For this review, take the finished solid that the model builds, in its own axes (mm). A direction names the side the tool comes from. Give positions to 0.01 mm unless a question says otherwise; leave off trailing zeros. Loops run counter-clockwise (first coordinate to the right, second up) from the corner with the lowest first, then second, coordinate; pieces in that order, holes last. Notation, with made-up numbers: (-9.5, 65) -> (19.5, 65) arc R18 cw to (19.5, 91) -> close; hole circle Ø5 at (58, -4.5). An arc over 180 degrees is marked (long way). Write each question's results on one line, items separated by ' | '. Start each with the question number.
```python
from build123d import *

# Parameters (mm, degrees)
SKETCH_R          = 2
PAD_DEPTH         = 26
POCKET_DEPTH      = 12
POCKET_DEPTH_BACK = -12
POCKET001_DEPTH   = 4
CHAMFER_SIZE      = 3
SKETCH003_R       = 3
POCKET002_DEPTH   = 26
SKETCH004_R       = 6.75
POCKET003_DEPTH   = 5
FILLET_R          = 4.5
FILLET001_R       = 5
CHAMFER001_SIZE   = 0.5


with BuildPart() as part:
    # Sketch → Pad (new body)
    with BuildSketch(Plane.XY):
        with BuildLine():
            ThreePointArc((1e-06, -3.5), (3.416335, -0.760696), (1.485025, 3.169337))
            Line((-45.1066, 25), (1.485025, 3.169337))
            Line((-45.1066, 7.106602), (-45.1066, 25))
            Line((-34.499999, -3.5), (-45.1066, 7.106602))
            Line((1e-06, -3.5), (-34.499999, -3.5))
        make_face()
        Circle(SKETCH_R, mode=Mode.SUBTRACT)
    extrude(amount=PAD_DEPTH)

    # Sketch001 (on DatumPlane) → Pocket (cut, two sides)
    with BuildSketch(Plane.XY.offset(13)) as pocket_sk:
        Polygon((-60, 17), (-10, 17), (-60, 55), align=None)
    extrude(amount=-POCKET_DEPTH, mode=Mode.SUBTRACT)
    extrude(pocket_sk.sketch, amount=-POCKET_DEPTH_BACK, mode=Mode.SUBTRACT)

    # Sketch002 → Pocket001 (cut)
    with BuildSketch(Plane.XY):
        Polygon((-19.5, -3.5), (-30.106602, 7.106602), (-45.106602, 7.106602), (-34.5, -3.5), align=None)
    extrude(amount=POCKET001_DEPTH, mode=Mode.SUBTRACT)

    # Chamfer
    chamfer_edges = [part.edges().sort_by_distance(p)[0] for p in [
        (-36.569686, 17, 1),
        (-36.569686, 17, 25),
    ]]
    chamfer(chamfer_edges, length=CHAMFER_SIZE)

    # Sketch003 → Pocket002 (cut)
    with BuildSketch(Plane.XY):
        with Locations((-32.5, 1.5)):
            Circle(SKETCH003_R)
    extrude(amount=POCKET002_DEPTH, mode=Mode.SUBTRACT)

    # Sketch004 → Pocket003 (cut)
    with BuildSketch(Plane.XZ):
        with Locations((-20, 13)):
            Circle(SKETCH004_R)
    extrude(amount=POCKET003_DEPTH, mode=Mode.SUBTRACT)

    # Fillet
    fillet_edges = [part.edges().sort_by_distance(p)[0] for p in [
        (-45.1066, 17, 13),
        (-45.1066, 18.5, 2.5),
        (-45.1066, 18.5, 23.5),
        (-31.234114, 18.5, 23.5),
        (-31.234114, 18.5, 2.5),
    ]]
    fillet(fillet_edges, radius=FILLET_R)

    # Fillet001
    fillet001_edges = [part.edges().sort_by_distance(p)[0] for p in [
        (-45.1066, 25, 0.5),
        (-45.1066, 25, 25.5),
    ]]
    fillet(fillet001_edges, radius=FILLET001_R)

    # Chamfer001
    chamfer001_edges = [part.edges().sort_by_distance(p)[0] for p in [
        (-39.803299, 1.803301, 26),
        (-18.250068, 12.416282, 26),
    ]]
    chamfer(chamfer001_edges, length=CHAMFER001_SIZE)


solid = part.part
```
1. We need section A-A (x = -1). Write out the cut boundary in (y, z).
2. For pin 1 Ø10 at (x, z) = (-34, 10.5) entering from +Y; pin 2 Ø5 at (y, z) = (17, 19.5) entering from +X; pin 3 Ø10 at (y, z) = (9, 4) entering from +X, all flat-tipped, find the tip position at first contact; note any pin that passes through.
3. We need section C-C (x = -20). Write out the cut boundary in (y, z).
4. We need section D-D (y = 10.5). Write out the cut boundary in (x, z), plus the area to 3 significant figures.
5. We need section B-B (z = 21.5). Write out the cut boundary in (x, y).
6. Wall thickness on L1, parallel to Z at x = -20, y = -2.75; L2, parallel to Y at x = -32.5, z = 10; L3, parallel to X at y = -1.75, z = 8.25: over which ranges is each line inside the solid? List them lowest first.
7. Machinability: for faces 4 (the flat face through (-39.55, 1.9, 25.75)), 5 (the cylindrical face through (-43.82, 15.65, 12.85)), 6 (the flat face through (-37, 18, 23)), 7 (the flat face through (-29.6, 3.1, 4)), 8 (the cylindrical face through (-42.73, 21.39, 0.51)), which of the approach directions +Z, -Z, +X, -X, +Y, -Y give a long, thin tool a straight path to every point of the face, cutting with its end or side? Answer none if there is none.
8. Draft analysis for pull direction X (two halves, no side actions). For faces 1 (the flat face through (-26, 7, 26)), 2 (the cylindrical face through (-35.5, 1.6, 14.8)), 3 (the flat face through (-25, 2, 2)), state which applies: released by +X, released by -X, zero draft, split by the parting line, or undercut.
Response:
1) outline: (-3.5, 0) -> (-1.73, 0) -> (-1.73, 26) -> (-3, 26) -> (-3.5, 25.5) -> close; (1.73, 0) -> (4.33, 0) -> (4.33, 25.5) -> (3.78, 26) -> (1.73, 26) -> close
2) pin 1: stops at y = 17 | pin 2: stops at x = -22.7 | pin 3: stops at x = -0.29
3) outline: (-3.5, 4) -> (-3, 4) -> (-3, 0) -> (13.24, 0) -> (13.24, 25.5) -> (12.68, 26) -> (-3, 26) -> (-3.5, 25.5) -> (-3.5, 19.75) -> (0, 19.75) -> (0, 6.25) -> (-3.5, 6.25) -> close
4) outline: (-45.11, 0) -> (-14.16, 0) -> (-14.16, 25.5) -> (-15.34, 26) -> (-44.61, 26) -> (-45.11, 25.5) -> close | area: 804 mm2
5) outline: (-45.11, 7.11) -> (-34.5, -3.5) -> (0, -3.5) arc R3.5 ccw to (1.49, 3.17) -> (-28.03, 17) -> (-40.61, 17) arc R4.5 ccw to (-45.11, 12.5) -> close; hole circle Ø6 at (-32.5, 1.5); hole circle Ø4 at (0, 0)
6) L1: z = 0 to 6.25, 19.75 to 26 | L2: y = -3.5 to -1.5, 4.5 to 17 | L3: x = -36.25 to -24.8, -15.2 to -0.97, 0.97 to 3.03
7) face 4: +Z, -X, -Y | face 5: -X, +Y | face 6: +X, -X, +Y | face 7: -Z, -X, -Y | face 8: +Z, -Z, +Y
8) face 1: zero draft | face 2: undercut | face 3: released by -X
